The listing builds one solid part. Answer for the finished solid, in the listing's coordinates (mm). A direction names the side the tool comes from. Coordinates: 2 decimals unless noted, no trailing zeros. Write each loop counter-clockwise with the first axis right and the second up, starting at its lowest first coordinate (ties: lowest second). Pieces come first, ordered by that corner, then holes. Notation, with made-up numbers: M 86,24.25 L 104,24.25 A14 cw 104,38.25 Z; hole C -8,2.25 d1. An arc over 180 degrees is marked long. Put each result on its own line as item: value. Start each with the question number.
```python
from build123d import *

# Parameters (mm, degrees)
SKETCH1_R                               = 11
BOSS_EXTRUDE1_DEPTH                     = 2
SKETCH2_R                               = 8
BOSS_EXTRUDE2_DEPTH                     = 14
CBORE_FOR_M5_HEX_HEAD_BOLT1_D           = 3
CBORE_FOR_M5_HEX_HEAD_BOLT1_CBORE_D     = 6
CBORE_FOR_M5_HEX_HEAD_BOLT1_CBORE_DEPTH = 3


with BuildPart() as part:
    # Sketch1 → Boss-Extrude1 (new body)
    with BuildSketch(Plane.XY):
        Circle(SKETCH1_R)
    extrude(amount=BOSS_EXTRUDE1_DEPTH)

    # Sketch2 → Boss-Extrude2 (add)
    with BuildSketch(Plane.XY.offset(2)):
        Circle(SKETCH2_R)
    extrude(amount=BOSS_EXTRUDE2_DEPTH)

    # CBORE for M5 Hex Head Bolt1 (through all)
    with Locations(Plane(origin=(0, 0, 0), x_dir=(-1, 0, 0), z_dir=(0, 0, -1))):
        with Locations((0, 0)):
            CounterBoreHole(CBORE_FOR_M5_HEX_HEAD_BOLT1_D / 2, CBORE_FOR_M5_HEX_HEAD_BOLT1_CBORE_D / 2, CBORE_FOR_M5_HEX_HEAD_BOLT1_CBORE_DEPTH)


solid = part.part
```
1) Given pin 1 Ø4 at (x, z) = (2.5, 9.5) entering from -Y; pin 2 Ø4 at (y, z) = (-9, 12.5) entering from +X; pin 3 Ø6 at (x, z) = (-2, 8.5) entering from +Y, each flat-ended and moving along its own axis, determine where each tip first touches the part or whether it passes through.
2) For faces 1 (the face through (-2.38, -10.74, 0.99)), 2 (the face through (-1.73, -7.81, 8.9)), 3 (the face through (-1.3, -1.3, 3)), determine the directions among +Z, -Z, +X, -X, +Y, -Y from which every point of the face is accessible in a straight line to the end or side of a thin tool.
3) A cutting plane is placed at A-A on x = 0. Write down the section's boundary in (y, z), then the cut area to 3 significant figures.
4) A cutting plane is placed at D-D on x = 4.25. Write down the section's boundary in (y, z), then the cut area to 3 significant figures.
5) A cutting plane is placed at C-C on z = 1.25. Write down the section's boundary in (x, y), then the cut area to 3 significant figures.
6) Straight lines are drawn through the part: probe 1 along Y at (x, z) = (0, 13); probe 2 along Z at (x, y) = (-8.5, -6); probe 3 along Y at (x, z) = (0.5, 5.75). For each, find the intervals that lie inside material, in ascending order.
Answers follow:
1. pin 1: stops at y = -7.98
1. pin 2: stops at x = 3.87
1. pin 3: stops at y = 8
2. face 1: +Z, -Z
2. face 2: +Z
2. face 3: -Z
3. outline: M -11,0 L -3,0 L -3,3 L -1.5,3 L -1.5,16 L -8,16 L -8,2 L -11,2 Z; M 1.5,3 L 3,3 L 3,0 L 11,0 L 11,2 L 8,2 L 8,16 L 1.5,16 Z
3. area: 211 mm²
4. outline: M -10.15,0 L 10.15,0 L 10.15,2 L 6.78,2 L 6.78,16 L -6.78,16 L -6.78,2 L -10.15,2 Z
4. area: 230 mm²
5. outline: C 0,0 d22; hole C 0,0 d6
5. area: 352 mm²
6. probe 1: y = -8 to -1.5, 1.5 to 8
6. probe 2: z = 0 to 2
6. probe 3: y = -7.98 to -1.41, 1.41 to 7.98
